Input: part model. Units: mm. Frame: model coordinates. A direction names the side the tool comes from. Give positions to 0.01 mm unless a question says otherwise; leave off trailing zeros. Return JSON: item names as keys, results as strings. Group by question number.
```python
from build123d import *

# Parameters (mm, degrees)
F1_DEPTH    = 50
F3_SIZE2    = 141.7820454904
F3_SIZE     = 25
F4_SIZE2    = 24.99999
F4_SIZE     = 189.893843
F5_SIZE2    = 141.782035
F5_SIZE     = 24.99999
F5_2_SIZE2  = 141.782035
F5_2_SIZE   = 24.99999
F6_T1_DEPTH = 477.1700191754
F7_T1_DEPTH = 506.6441108429
F8_SIZE2    = 25
F8_SIZE     = 93.3012701892
F8_2_SIZE2  = 24.99999
F8_2_SIZE   = 93.30126
F10_DEPTH   = 25


# Not quite as in the source:
# - a fillet or chamfer that OpenCascade refuses, or shapes differently, is made with other operations: its cross-section is extruded or revolved along the edge and cut away or added
# - a fillet or chamfer is up to 0.001 mm smaller than in the source, because OpenCascade refuses the exact size


with BuildPart() as f1:
    # F0 (on Front) → F1 (new body)
    with BuildSketch(Plane.XZ):
        Polygon((0, 200), (0, 0), (1000, 0), (1000, 1000), (800, 1000), (800, 720), (280, 720), (280, 200), align=None)
    extrude(amount=F1_DEPTH)


with BuildPart() as f1_1:
    # F2: moved
    add(f1.part.moved(Location((1592, 0, 0))))

    # F3
    f3_edges = [f1_1.edges().sort_by_distance(p)[0] for p in [
        (2592, 0, 500),
        (2092, 0, 0),
    ]]
    chamfer(f3_edges, length=F3_SIZE, length2=F3_SIZE2)

    # F4 (size 189.8938528181 and 25 in the source; OpenCascade refuses exactly that, so slightly less here)
    f4_edges = [f1_1.edges().sort_by_distance(p)[0] for p in [
        (2092, -50, 0),
        (2592, -50, 500),
    ]]
    f4_side = f1_1.faces().sort_by_distance((2210.680203, -50, 381.319797))[0]
    chamfer(f4_edges, length=F4_SIZE, length2=F4_SIZE2, reference=f4_side)

    # F5 (size 25 and 141.7820454904 in the source; OpenCascade refuses exactly that, so slightly less here)
    f5_edges = [f1_1.edges().sort_by_distance(p)[0] for p in [
        (2421.108977, 0, 1000),
        (2397.053079, -50, 1000),
    ]]
    f5_side = f1_1.faces().sort_by_distance((2461.151755, -23.287804, 1000))[0]
    chamfer(f5_edges, length=F5_SIZE, length2=F5_SIZE2, reference=f5_side)

    # F5#2 (size 25 and 141.7820454904 in the source; OpenCascade refuses exactly that, so slightly less here)
    f5_2_edges = [f1_1.edges().sort_by_distance(p)[0] for p in [
        (1592, 0, 170.891023),
        (1592, -50, 194.946922),
    ]]
    f5_2_side = f1_1.faces().sort_by_distance((1592, -23.287804, 130.848245))[0]
    chamfer(f5_2_edges, length=F5_2_SIZE, length2=F5_2_SIZE2, reference=f5_2_side)

    # F6: chamfer of 23 x 130.4394818512 on 2 edges, made by hand

    # F6_s2 → F6_t1 (cut)
    with BuildSketch(Plane.XY.offset(720)):
        Polygon((2522.4394818512, -50), (2392, -27), (2392, -50), align=None)
        Polygon((2392, -23), (2522.4394818512, 0), (2392, 0), align=None)
    extrude(amount=F6_T1_DEPTH, mode=Mode.SUBTRACT)

    # F7: chamfer of 25 x 141.7820454904 on 2 edges, made by hand

    # F7_s2 → F7_t1 (cut)
    with BuildSketch(Plane.YZ.offset(1365.3558891571)):
        Polygon((-25, 200), (0, 58.2179545096), (0, 200), align=None)
        Polygon((-50, 58.2179545096), (-25, 200), (-50, 200), align=None)
    extrude(amount=F7_T1_DEPTH, mode=Mode.SUBTRACT)

    # F8
    f8_edges = [f1_1.edges().sort_by_distance(p)[0] for p in [
        (1872, 0, 430.891023),
        (2161.108977, 0, 720),
    ]]
    f8_side = f1_1.faces().sort_by_distance((2161.108977, 0, 430.891023))[0]
    chamfer(f8_edges, length=F8_SIZE, length2=F8_SIZE2, reference=f8_side)

    # F8#2 (size 93.3012701892 and 25 in the source; OpenCascade refuses exactly that, so slightly less here)
    f8_2_edges = [f1_1.edges().sort_by_distance(p)[0] for p in [
        (1872, -50, 454.946922),
        (2137.053079, -50, 720),
    ]]
    f8_2_side = f1_1.faces().sort_by_distance((2137.053079, -50, 454.946921))[0]
    chamfer(f8_2_edges, length=F8_2_SIZE, length2=F8_2_SIZE2, reference=f8_2_side)

    # F9 (on face) → F10 (cut)
    with BuildSketch(Plane(origin=(76.0608571883, -431.3625565565, 0), x_dir=(-0.984807753, -0.1736481777, 0), z_dir=(-0.1736481777, 0.984807753, 0))):
        Polygon((-2346.6920852661, 742.4287796021), (-2347.2633361816, 957.3464989662), (-2383.4601961924, 957.3464989662), (-2383.4601961924, 742.4287796021), align=None)
    extrude(amount=-F10_DEPTH, mode=Mode.SUBTRACT)


solid = f1_1.part
```
Item 1: Material intervals for line 1 (Y direction, x = 2548, z = 106.5); line 2 (Y direction, x = 2200.5, z = 180), sorted ascending. Write a range as from..to.
Item 2: First-contact query: pin 1 Ø4.5 at (y, z) = (-25.5, 726) entering from -X. Flat tip, straight axial feed; report the tip coordinate or a pass-through.
Item 3: Reachability of faces 1 (the face through (2400.917, -28.572, 965.825)), 2 (the face through (2183.465, -12.675, 674.002)), 3 (the face through (2204, 0, 388)) from +Z, -Z, +X, -X, +Y, -Y: full face, straight path, thin tool, end or side. Return the list, or none.
Answer below:
{
 "1": {"line 1": "-30.79..-17.24", "line 2": "-48.7..0"},
 "2": {"pin 1": "x = 2392"},
 "3": {"face 1": "+Z, -X, -Y", "face 2": "+Z, -X, +Y", "face 3": "+Z, -Z, +X, -X, +Y"}
}
